Build history of the part. All positions in model axes, mm. A direction names the side the tool comes from. Round coordinates to 2 decimals unless told otherwise and drop trailing zeros. Loops run counter-clockwise (first coordinate to the right, second up) from the corner with the lowest first, then second, coordinate; pieces in that order, holes last. Notation, with made-up numbers: (-33, -31) - (-18, -31) arc R19 ccw to (-18, -5) - close; hole circle Ø2 at (32, -40). An arc over 180 degrees is marked (long way). Use a Markdown table: item, result.
from build123d import *

# Parameters (mm, degrees)
SKETCH_1_W        = 2
SKETCH_1_H        = 4
EXTRUDE_1_DEPTH   = 5.5
EXTRUDE_1_2_DEPTH = 5.5
SKETCH_1_3_W      = 4
SKETCH_1_3_H      = 4
EXTRUDE_2_DEPTH   = 1.5
FILLET_1_R        = 0.5


with BuildPart() as part:
    # Sketch 1 → Extrude 1 (new body)
    with BuildSketch(Plane(origin=(0, 0, 0), x_dir=(1, 0, 0), z_dir=(0, 1, 0))):
        with Locations((-3, 0)):
            Rectangle(SKETCH_1_W, SKETCH_1_H)
    extrude(amount=EXTRUDE_1_DEPTH)



with BuildPart() as body_2:
    # Sketch 1 → Extrude 1 2 (new body)
    with BuildSketch(Plane(origin=(0, 0, 0), x_dir=(1, 0, 0), z_dir=(0, 1, 0))):
        with Locations((3, 0)):
            Rectangle(SKETCH_1_W, SKETCH_1_H)
    extrude(amount=EXTRUDE_1_2_DEPTH)


with BuildPart() as part_1:
    add(part.part)

    add(body_2.part)  # Extrude 2 merges body 2
    # Sketch 1_3 → Extrude 2 (add)
    with BuildSketch(Plane(origin=(0, 0, 0), x_dir=(1, 0, 0), z_dir=(0, 1, 0))):
        Rectangle(SKETCH_1_3_W, SKETCH_1_3_H)
    extrude(amount=EXTRUDE_2_DEPTH)

    # Fillet 1
    fillet_1_edges = [part_1.edges().sort_by_distance(p)[0] for p in [
        (2, 1.5, 0),
        (-2, 1.5, 0),
    ]]
    fillet(fillet_1_edges, radius=FILLET_1_R)


solid = part_1.part
Q1. Cut at D-D, the plane x = 1.25. List the corners of the cut face in (y, z), plus the area to 3 significant figures.
Results found:
| item | result |
|---|---|
| outline | (0, -2) - (1.5, -2) - (1.5, 2) - (0, 2) - close |
| area | 6.00 mm2 |
Q2. Cut at A-A, the plane y = 1.6. List the corners of the cut face in (x, z), plus the area to 3 significant figures.
Results found:
| item | result |
|---|---|
| outline | (-4, -2) - (-1.8, -2) - (-1.8, 2) - (-4, 2) - close; (1.8, -2) - (4, -2) - (4, 2) - (1.8, 2) - close |
| area | 17.6 mm2 |
Q3. Which spindle directions (+Z, -Z, +X, -X, +Y, -Y) get a long thin tool onto all of the face, cutting with end or side? Do faces 1 (the face through (0, 1.5, 0)), 2 (the face through (0, 1, 2)). Say none if no direction does.
Results found:
| item | result |
|---|---|
| face 1 | +Z, -Z, +Y |
| face 2 | +Z, +X, -X, +Y, -Y |
Q4. Pull direction X, two halves, no side cores. Call faces 3 (the face through (-4, 3, 0)), 4 (the face through (-2, 4, 0)), 5 (the face through (0, 0, 0)): pulls with the +X half, pulls with the -X half, needs draft (parallel to the pull), parting line crosses it, or undercut.
Results found:
| item | result |
|---|---|
| face 3 | pulls with the -X half |
| face 4 | undercut |
| face 5 | needs draft |
Q5. Drop a flat-ended pin along its axis: pin 1 (2 mm diameter, centred on x = -0.5, z = -1, fed in from +Y). Give the stop position or say it passes through.
Results found:
| item | result |
|---|---|
| pin 1 | stops at y = 1.5 |
Q6. Cut at C-C, the plane y = 4.55. List the corners of the cut face in (x, z).
Results found:
| item | result |
|---|---|
| outline | (-4, -2) - (-2, -2) - (-2, 2) - (-4, 2) - close; (2, -2) - (4, -2) - (4, 2) - (2, 2) - close |
Q7. Probe line 1 (X direction, y = 4.4, z = 1.5); line 2 (Y direction, x = 0, z = -0.2); line 3 (Y direction, x = -1.75, z = 1.75). List the from-to ranges inside material, lowest first.
Results found:
| item | result |
|---|---|
| line 1 | x = -4 to -2, 2 to 4 |
| line 2 | y = 0 to 1.5 |
| line 3 | y = 0 to 1.57 |
Q8. Cut at B-B, the plane z = -0.05. List the corners of the cut face in (x, y), plus the area to 3 significant figures.
Results found:
| item | result |
|---|---|
| outline | (-4, 0) - (4, 0) - (4, 5.5) - (2, 5.5) - (2, 2) arc R0.5 cw to (1.5, 1.5) - (-1.5, 1.5) arc R0.5 cw to (-2, 2) - (-2, 5.5) - (-4, 5.5) - close |
| area | 28.1 mm2 |
